Here's how the part is built. I have some questions about the finished solid (model axes, mm). A direction names the side the tool comes from. Coordinates: 2 decimals unless noted, no trailing zeros. Write each loop counter-clockwise with the first axis right and the second up, starting at its lowest first coordinate (ties: lowest second). Pieces come first, ordered by that corner, then holes.
Item 1: I want a section at B-B (z = 8). Please give me the cut outline in (x, y), and give its area (3 significant figures).
Item 2: If we mould it in two halves opening along Y, with no side actions, what happens to faces 1 (the face through (2, -7, 14)), 2 (the face through (0, 31, 0))? For each: pulls with the +Y half, pulls with the -Y half, needs draft (parallel to the pull), parting line crosses it, or undercut.
Item 3: I want a section at D-D (z = -0.5). Please give me the cut outline in (x, y), and give its area (3 significant figures).
Item 4: I want a section at A-A (y = 0). Please give me the cut outline in (x, z).
Item 5: I want a section at C-C (x = 11.25). Please give me the cut outline in (y, z).
Item 6: Please list where these lines run through material, in increasing order: line 1 (Z direction, x = 1, y = 12); line 2 (Z direction, x = 5.25, y = 0); line 3 (Y direction, x = 5, z = -20).
Item 7: I'm going to push flat-ended pins straight in: P1, Ø0.9, axis at x = 6, z = 15.5, coming from the +Y side; P2, Ø1.1, axis at x = 8.5, z = -17.5, coming from the -Y side; P3, Ø1.1, axis at y = 7, z = -15, coming from the +X side; P4, Ø3, axis at x = 9.5, y = 10, coming from the -Z side. Where does each tip first touch, or does it pass through?
Item 8: For faces 3 (the face through (2.564, -6.88, 15.479)), 4 (the face through (2, 4, -14)), 5 (the face through (9, 0, 0)), which set-ups out of +Z, -Z, +X, -X, +Y, -Y let a thin tool reach every point of the face, with its end or its side?
from build123d import *

# Parameters (mm, degrees)
SKETCH_R             = 1.65
PAD_DEPTH            = 27.5
SKETCH001_R          = 7.65
POCKET_DEPTH         = 22.7
SKETCH002_W          = 2
SKETCH002_H          = 7
POCKET001_DEPTH      = 27.501
POCKET001_DEPTH_BACK = -27.501
SKETCH003_W          = 18
SKETCH003_H          = 5
POCKET002_DEPTH      = 0.001
POCKET002_DEPTH_BACK = -17.501
SKETCH004_W          = 23.804039
SKETCH004_H          = 32
POCKET003_DEPTH      = 27.501
POCKET003_DEPTH_BACK = -27.501
SKETCH005_W          = 7
SKETCH005_H          = 12
POCKET004_DEPTH      = 17.501
POCKET005_DEPTH      = 3
SKETCH007_W          = 24.471905
SKETCH007_H          = 61.781853
POCKET006_DEPTH      = 27.501
POCKET006_DEPTH_BACK = -27.501
SKETCH008_R          = 1.65
POCKET007_DEPTH      = 12.001
POCKET008_DEPTH      = 3
SKETCH010_W          = 7
SKETCH010_H          = 1
POCKET009_DEPTH      = 1


with BuildPart() as part:
    # Sketch → Pad (new body, symmetric)
    with BuildSketch(Plane.XY):
        with BuildLine():
            Line((0, 32.5), (5, 32.5))
            Line((5, 32.5), (17.5, 20))
            Line((17.5, 20), (17.5, -20))
            Line((17.5, -20), (5, -32.5))
            Line((5, -32.5), (0, -32.5))
            Line((0, -26.5), (0, -32.5))
            ThreePointArc((0, -26.5), (4, -22.5), (0, -18.5))
            Line((0, 18.5), (0, -18.5))
            ThreePointArc((0, 18.5), (4, 22.5), (0, 26.5))
            Line((0, 32.5), (0, 26.5))
        make_face()
        with Locations((5, 5.5)):
            Circle(SKETCH_R, mode=Mode.SUBTRACT)
        with Locations((5, -5.5)):
            Circle(SKETCH_R, mode=Mode.SUBTRACT)
    extrude(amount=PAD_DEPTH, both=True)

    # Sketch001 → Pocket (cut, symmetric)
    with BuildSketch(Plane.XY):
        with Locations((0, 22.5)):
            Circle(SKETCH001_R)
        with Locations((0, -22.5)):
            Circle(SKETCH001_R)
    extrude(amount=POCKET_DEPTH, both=True, mode=Mode.SUBTRACT)

    # Sketch002 → Pocket001 (cut, two sides)
    with BuildSketch(Plane.XY) as pocket001_sk:
        with Locations((0, 5.5)):
            Rectangle(SKETCH002_W, SKETCH002_H)
        with Locations((0, -5.5)):
            Rectangle(SKETCH002_W, SKETCH002_H)
    extrude(amount=-POCKET001_DEPTH, mode=Mode.SUBTRACT)
    extrude(pocket001_sk.sketch, amount=-POCKET001_DEPTH_BACK, mode=Mode.SUBTRACT)

    # Sketch003 → Pocket002 (cut, two sides)
    with BuildSketch(Plane.YZ) as pocket002_sk:
        with Locations((0, 25)):
            Rectangle(SKETCH003_W, SKETCH003_H)
        with Locations((0, -25)):
            Rectangle(SKETCH003_W, SKETCH003_H)
    extrude(amount=-POCKET002_DEPTH, mode=Mode.SUBTRACT)
    extrude(pocket002_sk.sketch, amount=-POCKET002_DEPTH_BACK, mode=Mode.SUBTRACT)

    # Sketch004 → Pocket003 (cut, two sides)
    with BuildSketch(Plane.XY) as pocket003_sk:
        with Locations((20.902019, 0)):
            Rectangle(SKETCH004_W, SKETCH004_H)
    extrude(amount=-POCKET003_DEPTH, mode=Mode.SUBTRACT)
    extrude(pocket003_sk.sketch, amount=-POCKET003_DEPTH_BACK, mode=Mode.SUBTRACT)

    # Sketch005 → Pocket004 (cut, through all)
    with BuildSketch(Plane.YZ):
        with Locations((-5.5, 8)):
            Rectangle(SKETCH005_W, SKETCH005_H)
        with Locations((-5.5, -8)):
            Rectangle(SKETCH005_W, SKETCH005_H)
        with Locations((5.5, 8)):
            Rectangle(SKETCH005_W, SKETCH005_H)
        with Locations((5.5, -8)):
            Rectangle(SKETCH005_W, SKETCH005_H)
    extrude(amount=POCKET004_DEPTH, mode=Mode.SUBTRACT)

    # Sketch006 (on DatumPlane) → Pocket005 (cut)
    with BuildSketch(Plane.XY.offset(14)):
        Polygon((8.233162, 5.5), (6.616581, 8.3), (3.383419, 8.3), (1.766838, 5.5), (3.383419, 2.7), (6.616581, 2.7), align=None)
        Polygon((8.233162, -5.5), (6.616581, -2.7), (3.383419, -2.7), (1.766838, -5.5), (3.383419, -8.3), (6.616581, -8.3), align=None)
    extrude(amount=POCKET005_DEPTH, mode=Mode.SUBTRACT)

    # Sketch007 → Pocket006 (cut, two sides)
    with BuildSketch(Plane.XY) as pocket006_sk:
        with Locations((24.235952, 0.497813)):
            Rectangle(SKETCH007_W, SKETCH007_H)
    extrude(amount=-POCKET006_DEPTH, mode=Mode.SUBTRACT)
    extrude(pocket006_sk.sketch, amount=-POCKET006_DEPTH_BACK, mode=Mode.SUBTRACT)

    # Sketch008 → Pocket007 (cut, through all)
    with BuildSketch(Plane.YZ):
        with Locations((12, 18)):
            Circle(SKETCH008_R)
        with Locations((-12, 18)):
            Circle(SKETCH008_R)
        with Locations((0, 18)):
            Circle(SKETCH008_R)
        with Locations((0, -18)):
            Circle(SKETCH008_R)
        with Locations((-12, -18)):
            Circle(SKETCH008_R)
        with Locations((12, -18)):
            Circle(SKETCH008_R)
    extrude(amount=POCKET007_DEPTH, mode=Mode.SUBTRACT)

    # Sketch009 (on DatumPlane) → Pocket008 (cut)
    with BuildSketch(Plane.XY.offset(-14)):
        Polygon((3.383419, 2.7), (6.616581, 2.7), (8.233162, 5.5), (6.616581, 8.3), (3.383419, 8.3), (1.766838, 5.5), align=None)
        Polygon((8.233162, -5.5), (6.616581, -2.7), (3.383419, -2.7), (1.766838, -5.5), (3.383419, -8.3), (6.616581, -8.3), align=None)
    extrude(amount=-POCKET008_DEPTH, mode=Mode.SUBTRACT)

    # Sketch010 (on DatumPlane) → Pocket009 (cut)
    with BuildSketch(Plane.YZ.offset(9)):
        with Locations((-5.5, 15.25)):
            Rectangle(SKETCH010_W, SKETCH010_H)
        with Locations((-5.5, 17.25)):
            Rectangle(SKETCH010_W, SKETCH010_H)
        with Locations((-5.5, 19.25)):
            Rectangle(SKETCH010_W, SKETCH010_H)
        with Locations((-5.5, 21.25)):
            Rectangle(SKETCH010_W, SKETCH010_H)
        with Locations((5.5, 15.25)):
            Rectangle(SKETCH010_W, SKETCH010_H)
        with Locations((5.5, 17.25)):
            Rectangle(SKETCH010_W, SKETCH010_H)
        with Locations((5.5, 19.25)):
            Rectangle(SKETCH010_W, SKETCH010_H)
        with Locations((5.5, 21.25)):
            Rectangle(SKETCH010_W, SKETCH010_H)
        with Locations((-5.5, -21.25)):
            Rectangle(SKETCH010_W, SKETCH010_H)
        with Locations((-5.5, -19.25)):
            Rectangle(SKETCH010_W, SKETCH010_H)
        with Locations((-5.5, -17.25)):
            Rectangle(SKETCH010_W, SKETCH010_H)
        with Locations((-5.5, -15.25)):
            Rectangle(SKETCH010_W, SKETCH010_H)
        with Locations((5.5, -21.25)):
            Rectangle(SKETCH010_W, SKETCH010_H)
        with Locations((5.5, -19.25)):
            Rectangle(SKETCH010_W, SKETCH010_H)
        with Locations((5.5, -17.25)):
            Rectangle(SKETCH010_W, SKETCH010_H)
        with Locations((5.5, -15.25)):
            Rectangle(SKETCH010_W, SKETCH010_H)
    extrude(amount=-POCKET009_DEPTH, mode=Mode.SUBTRACT)


solid = part.part
Answer:
1. outline: (0, -32.5) - (5, -32.5) - (12, -25.5) - (12, -16) - (9, -16) - (9, -9) - (0, -9) - (0, -14.85) arc R7.65 cw to (0, -30.15) - close; (0, -2) - (9, -2) - (9, 2) - (0, 2) - close; (0, 9) - (9, 9) - (9, 16) - (12, 16) - (12, 25.5) - (5, 32.5) - (0, 32.5) - (0, 30.15) arc R7.65 cw to (0, 14.85) - close
1. area: 325 mm2
2. face 1: undercut
2. face 2: needs draft
3. outline: (0, -32.5) - (5, -32.5) - (12, -25.5) - (12, -16) - (9, -16) - (9, 16) - (12, 16) - (12, 25.5) - (5, 32.5) - (0, 32.5) - (0, 30.15) arc R7.65 cw to (0, 14.85) - (0, 9) - (1, 9) - (1, 2) - (0, 2) - (0, -2) - (1, -2) - (1, -9) - (0, -9) - (0, -14.85) arc R7.65 cw to (0, -30.15) - close; hole circle Ø3.3 at (5, -5.5); hole circle Ø3.3 at (5, 5.5)
3. area: 420 mm2
4. outline: (0, -22.5) - (9, -22.5) - (9, -19.65) - (0, -19.65) - close; (0, -16.35) - (9, -16.35) - (9, 16.35) - (0, 16.35) - close; (0, 19.65) - (9, 19.65) - (9, 22.5) - (0, 22.5) - close
5. outline: (-26.25, -27.5) - (-16, -27.5) - (-16, 27.5) - (-26.25, 27.5) - close; (16, -27.5) - (26.25, -27.5) - (26.25, 27.5) - (16, 27.5) - close
6. line 1: z = -27.5 to -19.65, -16.35 to 16.35, 19.65 to 27.5
6. line 2: z = -22.5 to -19.65, -16.35 to 16.35, 19.65 to 22.5
6. line 3: y = -32.5 to -28.29, -16.71 to -7.15, -3.85 to 3.85, 7.15 to 16.71, 28.29 to 32.5
7. P1: stops at y = 31.95
7. P2: stops at y = -29.55
7. P3: stops at x = 9
7. P4: stops at z = -27.5
8. face 3: none
8. face 4: +X, -X
8. face 5: +Z, -Z, +X
